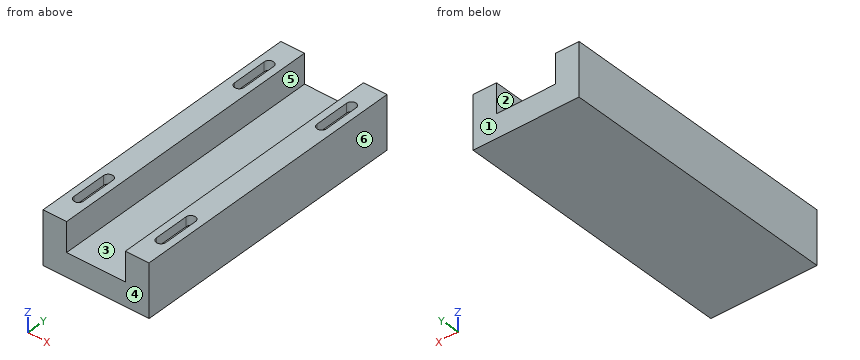
```python
from build123d import *

# Parameters (mm, degrees)
BOSS_EXTRUDE1_DEPTH  = 120
CUT_EXTRUDE1_DEPTH   = 4
MIRROR2_COPY_1_DEPTH = 4


with BuildPart() as part:
    # Sketch2 → Boss-Extrude1 (new body)
    with BuildSketch(Plane(origin=(0, 0, 0), x_dir=(1, 0, 0), z_dir=(0, 1, 0))):
        Polygon((0, 0), (-10, 0), (-10, 22.5), (35, 22.5), (35, 0), (25, 0), (25, 12.5), (0, 12.5), align=None)
    extrude(amount=BOSS_EXTRUDE1_DEPTH)

    # Sketch3 → Cut-Extrude1 (cut)
    with BuildSketch(Plane.XY):
        with BuildLine():
            Line((28, 108), (28, 93))
            ThreePointArc((28, 93), (30, 91), (32, 93))
            Line((32, 93), (32, 108))
            ThreePointArc((32, 108), (30, 110), (28, 108))
        make_face()
    cut_extrude1 = extrude(amount=-CUT_EXTRUDE1_DEPTH, mode=Mode.SUBTRACT)

    # Mirror1: Cut-Extrude1 across plane
    add(cut_extrude1.mirror(Plane.ZY.offset(-12.5)), mode=Mode.SUBTRACT)

    # Mirror2: Cut-Extrude1 across plane
    add(cut_extrude1.mirror(Plane(origin=(0, 60, 0), x_dir=(0, 0, 1), z_dir=(0, -1, 0))), mode=Mode.SUBTRACT)

    # Mirror2 copy 1 sketch → Mirror2 copy 1 (cut)
    with BuildSketch(Plane(origin=(25, 120, 0), x_dir=(-1, 0, 0), z_dir=(0, 0, 1))):
        with BuildLine():
            Line((28, 108), (28, 93))
            ThreePointArc((28, 93), (30, 91), (32, 93))
            Line((32, 93), (32, 108))
            ThreePointArc((32, 108), (30, 110), (28, 108))
        make_face()
    extrude(amount=-MIRROR2_COPY_1_DEPTH, mode=Mode.SUBTRACT)


solid = part.part
```
Here's how the part is built. I have some questions about the finished solid (model axes, mm). Face numbers are marked on the shaded views. A direction names the side the tool comes from. Give positions to 0.01 mm unless a question says otherwise; leave off trailing zeros. Order: outer loops, then holes, each group sorted by start corner. A loop starts at its lowest first (then second) coordinate and runs counter-clockwise, first axis right, second up. Notation, with made-up numbers: M 24.5,-14 L 30.5,-14 A35 cw 30.5,19 Z; hole C 31,76 d10. An arc over 180 degrees is marked long. Use a Markdown table: item, result. Add a question column.
1. If we mould it in two halves opening along X, with no side actions, what happens to the marked faces 3, 4, 5 and 6? For each: +X half, -X half, draft (parallel to the pull), parting line (faces both ways), or undercut.
2. Suppose I cut it at A-A (z = -10.25). List the corners of the cut face in (x, y) for me.
3. On a 3-axis mill with a long thin cutter (end or side, diameter ignored), from which of +Z, -Z, +X, -X, +Y, -Y can I reach the whole of each face in a straight line? I mean the marked faces 1 and 2. Say none if no direction works.
4. Suppose I cut it at C-C (x = -5). List the corners of the cut face in (y, z) for me, and give its area (3 significant figures).
5. For pin 1 Ø1.2 at (x, y) = (-5.5, 99) entering from +Z; pin 2 Ø1 at (x, y) = (22.5, 102) entering from +Z, each with a flat end and sliding along its axis, tell me the tip position at first contact or that it passes through.
6. Suppose I cut it at B-B (y = 30.5). List the corners of the cut face in (x, z) for me.
7. Suppose I cut it at D-D (y = 97). List the corners of the cut face in (x, z) for me, and give its area (3 significant figures).
8. I need wall thicknesses on probe 1 along X at (y, z) = (57, -7.75); probe 2 along Z at (x, y) = (5, 95.5). Which ranges of each line are inside material? Lowest first, please. Write a range as from..to.
Results list:
| question | item | result |
|---|---|---|
| 1 | face 3 | undercut |
| 1 | face 4 | draft |
| 1 | face 5 | undercut |
| 1 | face 6 | +X half |
| 2 | outline | M -10,0 L 0,0 L 0,120 L -10,120 Z; M 25,0 L 35,0 L 35,120 L 25,120 Z |
| 3 | face 1 | +Z, -Z, +X, -X, +Y |
| 3 | face 2 | +Z, +Y, -Y |
| 4 | outline | M 0,-22.5 L 120,-22.5 L 120,0 L 110,0 L 110,-4 L 91,-4 L 91,0 L 29,0 L 29,-4 L 10,-4 L 10,0 L 0,0 Z |
| 4 | area | 2,550 mm² |
| 5 | pin 1 | stops at z = -4 |
| 5 | pin 2 | stops at z = -12.5 |
| 6 | outline | M -10,-22.5 L 35,-22.5 L 35,0 L 25,0 L 25,-12.5 L 0,-12.5 L 0,0 L -10,0 Z |
| 7 | outline | M -10,-22.5 L 35,-22.5 L 35,0 L 32,0 L 32,-4 L 28,-4 L 28,0 L 25,0 L 25,-12.5 L 0,-12.5 L 0,0 L -3,0 L -3,-4 L -7,-4 L -7,0 L -10,0 Z |
| 7 | area | 668 mm² |
| 8 | probe 1 | x = -10..0, 25..35 |
| 8 | probe 2 | z = -22.5..-12.5 |
